Answer from the drawing. Dimensions are ordinates in mm from the lowest x, y and z of the part. A direction names the side the tool comes from. Give positions to 0.01 mm unless a question says otherwise; leave off trailing zeros. Write each loop counter-clockwise with the first axis right and the second up, starting at its lowest first coordinate (ties: lowest second). Pieces come first, ordered by that corner, then holes.
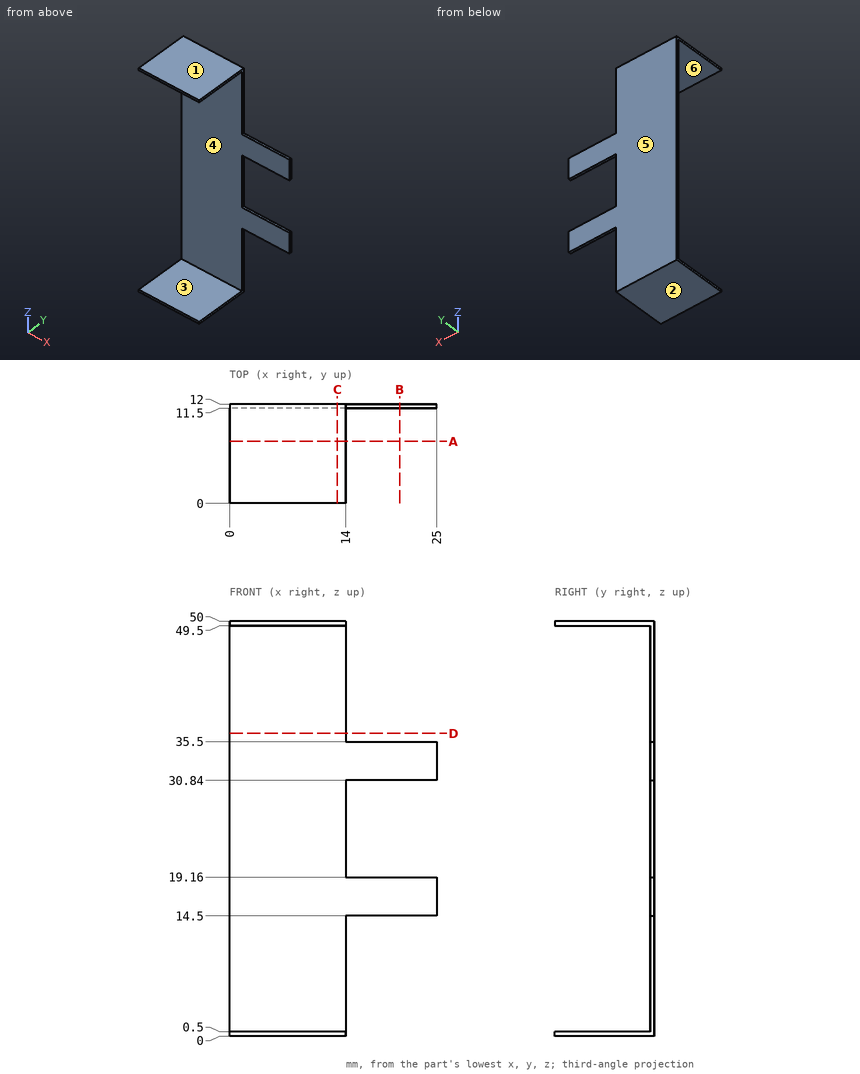
Item 1: A cutting plane is placed at B-B, the plane x = 20.5. Give the vertices of the cut face in (y, z), plus the area to 3 significant figures.
Conclusion:
outline: (11.5, 14.5) - (12, 14.5) - (12, 19.16) - (11.5, 19.16) - close; (11.5, 30.84) - (12, 30.84) - (12, 35.5) - (11.5, 35.5) - close
area: 4.66 mm2
Item 2: Determine the mould class of the marked faces 1, 2, 3 and 4 for opening direction Z: pulls with the +Z half, pulls with the -Z half, needs draft (parallel to the pull), parting line crosses it, or undercut.
Conclusion:
face 1: pulls with the +Z half
face 2: pulls with the -Z half
face 3: undercut
face 4: undercut
Item 3: Consider probe 1 along Z at (x, y) = (7.75, 9.5); probe 2 along Y at (x, z) = (9.5, 27.5). Determine where each line is inside the solid, lowest interval first.
Conclusion:
probe 1: z = 0 to 0.5, 49.5 to 50
probe 2: y = 11.5 to 12
Item 4: Which of the six approach directions +Z, -Z, +X, -X, +Y, -Y give full straight-line access (tool end or side, diameter ignored) to the marked faces 5 and 6?
Conclusion:
face 5: +Z, -Z, +X, -X, +Y
face 6: +X, -X, -Y
Item 5: A cutting plane is placed at A-A, the plane y = 7.5. Give the vertices of the cut face in (x, z), plus the area to 3 significant figures.
Conclusion:
outline: (0, 0) - (14, 0) - (14, 0.5) - (0, 0.5) - close; (0, 49.5) - (14, 49.5) - (14, 50) - (0, 50) - close
area: 14.0 mm2
Item 6: Each of these flat-tipped pins is pushed along its axis until it touches: P1, Ø0.6, axis at x = 17.5, y = 12, coming from the +Z side; P2, Ø0.6, axis at x = 20, y = 11.5, coming from the -Z side; P3, Ø12, axis at x = 4, z = 40, coming from the -Y side. Where does it stop, or does it pass through?
Conclusion:
P1: stops at z = 35.5
P2: stops at z = 14.5
P3: stops at y = 11.5
Item 7: A cutting plane is placed at D-D, the plane z = 36.5. Give the vertices of the cut face in (x, y).
Conclusion:
outline: (0, 11.5) - (14, 11.5) - (14, 12) - (0, 12) - close
Item 8: A cutting plane is placed at C-C, the plane x = 13. Give the vertices of the cut face in (y, z).
Conclusion:
outline: (0, 0) - (12, 0) - (12, 50) - (0, 50) - (0, 49.5) - (11.5, 49.5) - (11.5, 0.5) - (0, 0.5) - close
